Could you check a few things on this drawing? It's one solid part, dimensions in mm from its lowest x, y, z. A direction names the side the tool comes from. Round coordinates to 2 decimals unless told otherwise and drop trailing zeros. Loops run counter-clockwise (first coordinate to the right, second up) from the corner with the lowest first, then second, coordinate; pieces in that order, holes last. Notation, with made-up numbers: (26.25, 10.5) -> (79.25, 10.5) arc R33 ccw to (79.25, 45.5) -> close; hole circle Ø2 at (87.25, 88.5). An arc over 180 degrees is marked (long way). Write each question's results on one line, items separated by ' | '.
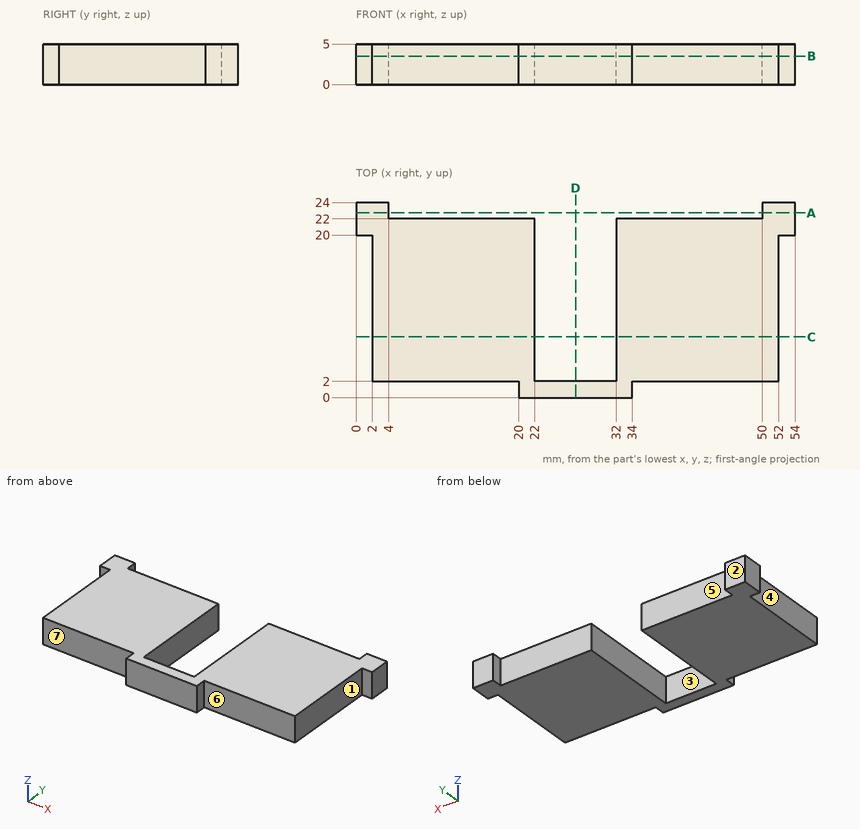
1) For the marked faces 5, 6 and 7, which set-ups out of +Z, -Z, +X, -X, +Y, -Y let a thin tool reach every point of the face, with its end or its side?
Model answer:
face 5: +Z, -Z, +Y | face 6: +Z, -Z, +X, -Y | face 7: +Z, -Z, -X, -Y
2) I want a section at D-D, the plane x = 27. Write out the boundary of the cut face in (y, z), plus the area to 3 significant figures.
Model answer:
outline: (0, 0) -> (2, 0) -> (2, 5) -> (0, 5) -> close | area: 10.0 mm2
3) I want a section at C-C, the plane y = 7.5. Write out the boundary of the cut face in (x, z).
Model answer:
outline: (2, 0) -> (22, 0) -> (22, 5) -> (2, 5) -> close; (32, 0) -> (52, 0) -> (52, 5) -> (32, 5) -> close
4) I want a section at A-A, the plane y = 22.75. Write out the boundary of the cut face in (x, z), plus the area to 3 significant figures.
Model answer:
outline: (0, 0) -> (4, 0) -> (4, 5) -> (0, 5) -> close; (50, 0) -> (54, 0) -> (54, 5) -> (50, 5) -> close | area: 40.0 mm2
5) I'm going to push flat-ended pins straight in: pin 1 (1 mm diameter, centred on y = 1, z = 2, fed in from -X); pin 2 (1 mm diameter, centred on x = 13.5, z = 2.5, fed in from +Y); pin 3 (2.5 mm diameter, centred on x = 24.5, z = 2, fed in from +Y); pin 4 (1 mm diameter, centred on x = 15.5, y = 5, fed in from -Z). Where does each tip first touch, or does it pass through?
Model answer:
pin 1: stops at x = 20 | pin 2: stops at y = 22 | pin 3: stops at y = 2 | pin 4: stops at z = 0
6) If we mould it in two halves opening along X, with no side actions, what happens to the marked faces 1, 2, 3 and 4? For each: released by +X, released by -X, zero draft, split by the parting line, or undercut.
Model answer:
face 1: released by +X | face 2: zero draft | face 3: undercut | face 4: released by -X
7) I need wall thicknesses on line 1 (X direction, y = 5, z = 2.6); line 2 (X direction, y = 23.25, z = 1.25); line 3 (X direction, y = 1.5, z = 4). Which ranges of each line are inside material? Lowest first, please.
Model answer:
line 1: x = 2 to 22, 32 to 52 | line 2: x = 0 to 4, 50 to 54 | line 3: x = 20 to 34
8) I want a section at B-B, the plane z = 3.5. Write out the boundary of the cut face in (x, y).
Model answer:
outline: (0, 20) -> (2, 20) -> (2, 2) -> (20, 2) -> (20, 0) -> (34, 0) -> (34, 2) -> (52, 2) -> (52, 20) -> (54, 20) -> (54, 24) -> (50, 24) -> (50, 22) -> (32, 22) -> (32, 2) -> (22, 2) -> (22, 22) -> (4, 22) -> (4, 24) -> (0, 24) -> close
